Design review of the part built by this model. Coordinates are the model's own, in mm. A direction names the side the tool comes from. Round coordinates to 2 decimals unless told otherwise and drop trailing zeros. Loops run counter-clockwise (first coordinate to the right, second up) from the corner with the lowest first, then second, coordinate; pieces in that order, holes last. Notation, with made-up numbers: (21.5, 10) - (43.5, 10) arc R12 cw to (43.5, 20) - close; hole circle Ø9 at (15.5, 62). An arc over 180 degrees is marked (long way). One line per question, with ' | ' between items. Start each with the question number.
from build123d import *

# Parameters (mm, degrees)
SKETCH1_W            = 57
SKETCH1_H            = 60.5
BOSS_EXTRUDE1_DEPTH  = 25
SKETCH2_W            = 42.7
SKETCH2_H            = 43.793176539
CUT_EXTRUDE1_DEPTH   = 72.396778639
SKETCH3_W            = 90
SKETCH3_H            = 48
BOSS_EXTRUDE2_DEPTH  = 8
SKETCH4_W            = 3.5
SKETCH4_H            = 13.5
CUT_EXTRUDE2_DEPTH   = 85.17392708
LPATTERN1_COUNT      = 2
LPATTERN1_PITCH      = 76
LPATTERN1_COUNT_DIR2 = 2
LPATTERN1_PITCH_DIR2 = 26
SKETCH5_R            = 2.1
CUT_EXTRUDE3_DEPTH   = 8


with BuildPart() as part:
    # Sketch1 → Boss-Extrude1 (new body)
    with BuildSketch(Plane.XY):
        with Locations((0, 30.25)):
            Rectangle(SKETCH1_W, SKETCH1_H)
    extrude(amount=BOSS_EXTRUDE1_DEPTH)

    # Sketch2 → Cut-Extrude1 (cut, through all)
    with BuildSketch(Plane.XY.offset(25)):
        with Locations((0, 40.74658827)):
            Rectangle(SKETCH2_W, SKETCH2_H)
    extrude(amount=-CUT_EXTRUDE1_DEPTH, mode=Mode.SUBTRACT)

    # Sketch3 → Boss-Extrude2 (add)
    with BuildSketch(Plane(origin=(0, 0, 0), x_dir=(1, 0, 0), z_dir=(0, 1, 0))):
        with Locations((0, -24)):
            Rectangle(SKETCH3_W, SKETCH3_H)
    extrude(amount=BOSS_EXTRUDE2_DEPTH)

    # Sketch4 → Cut-Extrude2 (cut, through all)
    with BuildSketch(Plane(origin=(0, 8, 0), x_dir=(1, 0, 0), z_dir=(0, 1, 0))):
        with Locations((-38, -10)):
            Rectangle(SKETCH4_W, SKETCH4_H)
    cut_extrude2 = extrude(amount=-CUT_EXTRUDE2_DEPTH, mode=Mode.SUBTRACT)

    # LPattern1: Cut-Extrude2 2 × 2
    with Locations(*[(i * LPATTERN1_PITCH, 0, j * LPATTERN1_PITCH_DIR2) for i in range(LPATTERN1_COUNT) for j in range(LPATTERN1_COUNT_DIR2) if (i, j) != (0, 0)]):
        add(cut_extrude2, mode=Mode.SUBTRACT)

    # Sketch5 → Cut-Extrude3 (cut)
    with BuildSketch(Plane(origin=(0, 60.5, 0), x_dir=(1, 0, 0), z_dir=(0, 1, 0))):
        with Locations(Location((-24.85, -12.5, 0), (0, 0, 270))):
            Circle(SKETCH5_R)
        with Locations(Location((24.85, -12.5, 0), (0, 0, 270))):
            Circle(SKETCH5_R)
    extrude(amount=-CUT_EXTRUDE3_DEPTH, mode=Mode.SUBTRACT)


solid = part.part
1. Take a section at B-B, the plane z = 40. Give the boundary of the cut face in (x, y).
2. Take a section at A-A, the plane y = 46.5. Give the boundary of the cut face in (x, z), then the cut area to 4 significant figures.
3. To check wall thickness, follow line 1 along X through (y, z) = (56, 12.5); line 2 along X through (y, z) = (6, 5.5); line 3 along Z through (x, y) = (-37, 3). State the ranges of each line that lie inside material, in increasing order.
4. Take a section at D-D, the plane z = 18. Give the boundary of the cut face in (x, y), then the cut area to 3 significant figures.
5. Take a section at C-C, the plane x = 37.5. Give the boundary of the cut face in (y, z).
6. Machinability: for faces 3 (the face through (0, 18.85, 13)), 4 (the face through (-1, 8, 29)), 5 (the face through (-38, 4, 3.25)), 6 (the face through (-22.768, 56.556, 12.227)), which of the approach directions +Z, -Z, +X, -X, +Y, -Y give a long, thin tool a straight path to every point of the face, cutting with its end or side? Answer none if there is none.
7. The part is to be moulded in two halves that separate along X. For faces 1 (the face through (-22.6, 60.5, 12.3)), 2 (the face through (-38, 4, 16.75)), say which applies: pulls with the +X half, pulls with the -X half, needs draft (parallel to the pull), parting line crosses it, or undercut.
8. Clearance check with flat-ended pins moving along their axes: P1, Ø1.8, axis at x = -37, y = 5, coming from the -Z side; P2, Ø2, axis at x = -24, z = 12, coming from the +Y side; P3, Ø2, axis at y = 28.5, z = 11.5, coming from the +X side; P4, Ø10, axis at x = 26, z = 42, coming from the +Y side. State where each tip first meets the part, or that it passes through.
Answer list:
1) outline: (-45, 0) - (-39.75, 0) - (-39.75, 8) - (-45, 8) - close; (-36.25, 0) - (36.25, 0) - (36.25, 8) - (-36.25, 8) - close; (39.75, 0) - (45, 0) - (45, 8) - (39.75, 8) - close
2) outline: (-28.5, 0) - (-21.35, 0) - (-21.35, 25) - (-28.5, 25) - close; (21.35, 0) - (28.5, 0) - (28.5, 25) - (21.35, 25) - close | area: 357.5 mm²
3) line 1: x = -28.5 to -26.95, -22.75 to -21.35, 21.35 to 22.75, 26.95 to 28.5 | line 2: x = -45 to -39.75, -36.25 to 36.25, 39.75 to 45 | line 3: z = 0 to 3.25, 16.75 to 29.25, 42.75 to 48
4) outline: (-45, 0) - (45, 0) - (45, 8) - (28.5, 8) - (28.5, 60.5) - (21.35, 60.5) - (21.35, 18.85) - (-21.35, 18.85) - (-21.35, 60.5) - (-28.5, 60.5) - (-28.5, 8) - (-45, 8) - close | area: 1,930 mm²
5) outline: (0, 0) - (8, 0) - (8, 3.25) - (0, 3.25) - close; (0, 16.75) - (8, 16.75) - (8, 29.25) - (0, 29.25) - close; (0, 42.75) - (8, 42.75) - (8, 48) - (0, 48) - close
6) face 3: +Z, -Z, +Y | face 4: +Z, +Y | face 5: +Y, -Y | face 6: +Y
7) face 1: needs draft | face 2: undercut
8) P1: stops at z = 0 | P2: stops at y = 52.5 | P3: stops at x = 28.5 | P4: stops at y = 8
